Could you check a few things on this model? Use its own coordinates, in mm. Face numbers are marked on the shaded views. A direction names the side the tool comes from. Give positions to 0.01 mm unless a question says otherwise; leave off trailing zeros. Loops run counter-clockwise (first coordinate to the right, second up) from the corner with the lowest first, then second, coordinate; pieces in that order, holes last. Notation, with made-up numbers: (-35.5, -30.75) -> (6.5, -30.75) arc R22 cw to (6.5, -7.75) -> close; hole circle Ø3 at (-39, 20.5). An arc over 180 degrees is marked (long way). Write each question's results on one line, items separated by ' | '. Start each with the question number.
Q1. If I drill on line 1 along X through (y, z) = (-97.5, -7.5); line 2 along X through (y, z) = (-114.5, 3); line 3 along Z through (x, y) = (17.5, -73), over which ranges is the centre line in solid material (lowest first)?
Q2. If we section it at B-B, the plane z = 0: List the corners of the cut face in (x, y) for me.
Q3. If we section it at C-C, the plane z = -60: List the corners of the cut face in (x, y) for me, plus the area to 3 significant figures.
Q4. Which directions (+Z, -Z, +X, -X, +Y, -Y) give clear straight access to the entire face, cutting with the end or side of a thin tool? Please do the marked faces 1, 2 and 3.
Q5. If we section it at D-D, the plane y = -21: List the corners of the cut face in (x, z) for me, plus the area to 3 significant figures.
Q6. We'd pull the mould along X, two halves only. Please class the marked faces 4 and 5: released by +X, released by -X, zero draft, split by the parting line, or undercut.
Q7. Will these pins go through, and if not, where does the flat tip stop? P1, Ø22.5, axis at y = -146.5, z = -53.5, coming from the +X side; P2, Ø1, axis at x = -37.5, y = -115, coming from the +Z side; P3, Ø5, axis at y = -37, z = -28.5, coming from the +X side; P4, Ø8, axis at x = -14.5, y = -99.5, coming from the +Z side.
Q8. If we section it at A-A, the plane x = 0: List the corners of the cut face in (y, z) for me.
from build123d import *

# Parameters (mm, degrees)
BOSS_EXTRUDE1_DEPTH      = 25
BOSS_EXTRUDE1_DEPTH_BACK = 25
SKETCH2_W                = 60
SKETCH2_H                = 40
BOSS_EXTRUDE7_REACH      = 242.299
BOSS_EXTRUDE8_REACH      = 251.036
SWEEP3_PROFILE_R         = 5


with BuildPart() as part:
    # Sketch2 → Boss-Extrude1 (new, two sides: drawn at the far end of the back side and taken through both)
    with BuildSketch(Plane.XY.offset(-BOSS_EXTRUDE1_DEPTH_BACK)):
        with BuildLine():
            Line((-28.9435, 0), (-45.651634272, 0))
            Line((-45.651634272, 0), (-64.220455689, -212.2426))
            Line((-64.220455689, -212.2426), (64.220455689, -212.2426))
            Line((64.220455689, -212.2426), (45.651634272, 0))
            Line((45.651634272, 0), (28.9435, 0))
            ThreePointArc((28.9435, 0), (0, -28.9435), (-28.9435, 0))
        make_face()
        with Locations((0, -105.527024802)):
            Rectangle(SKETCH2_W, SKETCH2_H, mode=Mode.SUBTRACT)
    extrude(amount=BOSS_EXTRUDE1_DEPTH + BOSS_EXTRUDE1_DEPTH_BACK)

    # Boss-Extrude7: up to this plane
    boss_extrude7_end = Plane(origin=(-45.651634272, 0, -25), z_dir=(-0.9961946980917452, 0.08715574274766147, 0))
    # Sketch58 → Boss-Extrude7 (add, up to the surface)
    with BuildSketch(Plane(origin=(-45.651634272, 0, 0), x_dir=(0, 0, -1), z_dir=(1, 0, 0)), mode=Mode.PRIVATE) as boss_extrude7_sk1:
        Polygon((25, -106.1213), (25, -212.2426), (70, -212.2426), align=None)
    boss_extrude7_tool1 = split(extrude(boss_extrude7_sk1.sketch, amount=-BOSS_EXTRUDE7_REACH, mode=Mode.PRIVATE), bisect_by=boss_extrude7_end, keep=Keep.BOTH, mode=Mode.PRIVATE)
    add(boss_extrude7_tool1.solids().sort_by_distance((-45.651634, -176.868833, -40))[0])
    # Sketch58 → Boss-Extrude7 (add, up to the surface)
    with BuildSketch(Plane(origin=(-45.651634272, 0, 0), x_dir=(0, 0, -1), z_dir=(1, 0, 0)), mode=Mode.PRIVATE) as boss_extrude7_sk2:
        Polygon((-25, -212.2426), (-70, -212.2426), (-25, -106.1213), align=None)
    boss_extrude7_tool2 = split(extrude(boss_extrude7_sk2.sketch, amount=-BOSS_EXTRUDE7_REACH, mode=Mode.PRIVATE), bisect_by=boss_extrude7_end, keep=Keep.BOTH, mode=Mode.PRIVATE)
    add(boss_extrude7_tool2.solids().sort_by_distance((-45.651634, -176.868833, 40))[0])

    # Boss-Extrude8: up to this plane
    boss_extrude8_end = Plane(origin=(45.651634272, 0, -25), z_dir=(0.9961946980917452, 0.08715574274766147, 0))
    # Sketch59 → Boss-Extrude8 (add, up to the surface)
    with BuildSketch(Plane(origin=(45.651634272, 0, 0), x_dir=(0, 0, -1), z_dir=(1, 0, 0)), mode=Mode.PRIVATE) as boss_extrude8_sk1:
        Polygon((25, -106.1213), (25, -212.2426), (70, -212.2426), align=None)
    boss_extrude8_tool1 = split(extrude(boss_extrude8_sk1.sketch, amount=BOSS_EXTRUDE8_REACH, mode=Mode.PRIVATE), bisect_by=boss_extrude8_end, keep=Keep.BOTH, mode=Mode.PRIVATE)
    add(boss_extrude8_tool1.solids().sort_by_distance((45.651634, -176.868833, -40))[0])
    # Sketch59 → Boss-Extrude8 (add, up to the surface)
    with BuildSketch(Plane(origin=(45.651634272, 0, 0), x_dir=(0, 0, -1), z_dir=(1, 0, 0)), mode=Mode.PRIVATE) as boss_extrude8_sk2:
        Polygon((-25, -212.2426), (-70, -212.2426), (-25, -106.1213), align=None)
    boss_extrude8_tool2 = split(extrude(boss_extrude8_sk2.sketch, amount=BOSS_EXTRUDE8_REACH, mode=Mode.PRIVATE), bisect_by=boss_extrude8_end, keep=Keep.BOTH, mode=Mode.PRIVATE)
    add(boss_extrude8_tool2.solids().sort_by_distance((45.651634, -176.868833, 40))[0])



with BuildPart() as body_2:
    # Sketch60 → Revolve9 (revolve)
    with BuildSketch(Plane.XY):
        with BuildLine():
            Line((0, -117.527024802), (0, -93.527024802))
            ThreePointArc((0, -93.527024802), (-12, -105.527024802), (0, -117.527024802))
        make_face()
    revolve(axis=Axis((0, 0, 0), (0, -1, 0)))


with BuildPart() as part_1:
    add(part.part)

    add(body_2.part)  # Sweep3 merges body 2
    # Sweep3: sweep along a path in Sketch62
    with BuildLine(Plane.XY) as sweep3_path:
        Line((30, -105.527024802), (-30, -105.527024802))
    # Sweep3 profile (on start of the path) → Sweep3 (sweep)
    with BuildSketch(Plane(origin=(30, -105.527024802, 0), x_dir=(0, 0, -1), z_dir=(-1, 0, 0))):
        Circle(SWEEP3_PROFILE_R)
    sweep(path=sweep3_path.line)


solid = part_1.part
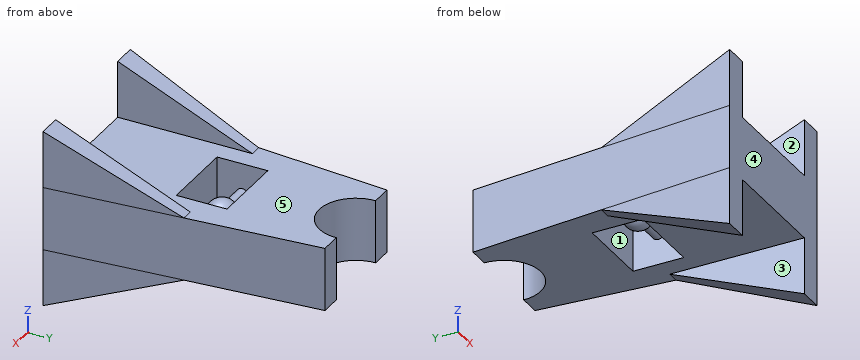
Final values:
1) line 1: x = -54.18 to -30, -4.83 to 4.83, 30 to 54.18 | line 2: x = -55.67 to -30, -7.38 to 7.38, 30 to 55.67 | line 3: z = -25 to 25
2) outline: (-64.22, -212.24) -> (64.22, -212.24) -> (45.65, 0) -> (28.94, 0) arc R28.94 cw to (-28.94, 0) -> (-45.65, 0) -> close; hole (-30, -125.53) -> (30, -125.53) -> (30, -110.53) -> (10.91, -110.53) arc R12 cw to (-10.91, -110.53) -> (-30, -110.53) -> close; hole (-30, -100.53) -> (-10.91, -100.53) arc R12 cw to (10.91, -100.53) -> (30, -100.53) -> (30, -85.53) -> (-30, -85.53) -> close
3) outline: (-64.22, -212.24) -> (-45.65, -212.24) -> (-45.65, -188.66) -> (-62.16, -188.66) -> close; (45.65, -212.24) -> (64.22, -212.24) -> (62.16, -188.66) -> (45.65, -188.66) -> close | area: 827 mm²
4) face 1: +Z, -Z | face 2: +Z, +Y, -Y | face 3: -Z, +Y, -Y
5) outline: (-47.49, -25) -> (-19.92, -25) -> (-19.92, 25) -> (-47.49, 25) -> close; (19.92, -25) -> (47.49, -25) -> (47.49, 25) -> (19.92, 25) -> close | area: 2,760 mm²
6) face 4: zero draft | face 5: undercut
7) P1: stops at x = 59.16 | P2: stops at z = 25 | P3: passes through | P4: stops at z = 4.57
8) outline: (-212.24, -25) -> (-125.53, -25) -> (-125.53, 25) -> (-212.24, 25) -> close; circle Ø24 at (-105.53, 0); (-85.53, -25) -> (-28.94, -25) -> (-28.94, 25) -> (-85.53, 25) -> close
